```python
from build123d import *

# Parameters (mm, degrees)
BOSS_EXTRUDE1_DEPTH  = 19.05
BOSS_EXTRUDE2_DEPTH  = 6.35
M6_CLEARANCE_HOLE1_D = 6.4
FILLET1_R            = 1


with BuildPart() as part:
    # Sketch1 → Boss-Extrude1 (new body)
    with BuildSketch(Plane(origin=(0, 0, 0), x_dir=(1, 0, 0), z_dir=(0, 1, 0))):
        with BuildLine():
            Line((-7.566372975, 10.2), (7.566372975, 10.2))
            ThreePointArc((7.566372975, 10.2), (12.7, 0), (7.566372975, -10.2))
            Line((7.566372975, -10.2), (-7.566372975, -10.2))
            ThreePointArc((-7.566372975, -10.2), (-12.7, 0), (-7.566372975, 10.2))
        make_face()
    extrude(amount=BOSS_EXTRUDE1_DEPTH)

    # Sketch1<4> → Boss-Extrude2 (add)
    with BuildSketch(Plane(origin=(0, 0, 0), x_dir=(1, 0, 0), z_dir=(0, 1, 0))):
        with BuildLine():
            Line((13.919410907, 37.5), (-13.919410907, 37.5))
            ThreePointArc((-13.919410907, 37.5), (-28.284271247, 28.284271247), (-37.5, 13.919410907))
            Line((-37.5, 13.919410907), (-37.5, -13.919410907))
            ThreePointArc((-37.5, -13.919410907), (-28.284271247, -28.284271247), (-13.919410907, -37.5))
            Line((-13.919410907, -37.5), (13.919410907, -37.5))
            ThreePointArc((13.919410907, -37.5), (28.284271247, -28.284271247), (37.5, -13.919410907))
            Line((37.5, -13.919410907), (37.5, 13.919410907))
            ThreePointArc((37.5, 13.919410907), (28.284271247, 28.284271247), (13.919410907, 37.5))
        make_face()
    extrude(amount=-BOSS_EXTRUDE2_DEPTH)

    # M6 Clearance Hole1 (through all)
    with Locations(Plane(origin=(-30, 0, 0), x_dir=(0, 0, 1), z_dir=(0, 1, 0))):
        with Locations((0, 0), (-25.980762114, 15), (-25.980762114, 45), (0, 60), (25.980762114, 45), (25.980762114, 15)):
            Hole(M6_CLEARANCE_HOLE1_D / 2)

    # Fillet1
    fillet1_edges = [part.edges().sort_by_distance(p)[0] for p in [
        (-7.566372975, 9.525, 10.2),
        (-7.566372975, 9.525, -10.2),
        (7.566372975, 9.525, -10.2),
        (7.566372975, 9.525, 10.2),
    ]]
    fillet(fillet1_edges, radius=FILLET1_R)


solid = part.part
```
Model file for the job. Use its own axes, mm. A direction names the side the tool comes from. Coordinates: 2 decimals unless noted, no trailing zeros. Write each loop counter-clockwise with the first axis right and the second up, starting at its lowest first coordinate (ties: lowest second). Pieces come first, ordered by that corner, then holes. Notation, with made-up numbers: (37.5, 37.5) - (83.5, 37.5) arc R17 ccw to (83.5, 43.5) - close; hole circle Ø9 at (42.25, 16). An arc over 180 degrees is marked (long way). One line per item, written item: value. Start each with the question number.
1. Tool access for faces 4 (the cylindrical face through (12.7, 9.4, -0.2)), 5 (the cylindrical face through (-12.7, 9.4, 0.2)), 6 (the flat face through (0, 9, 10.2)), 7 (the flat face through (0, 9, -10.2)): list every direction of +Z, -Z, +X, -X, +Y, -Y with a clear straight run to the whole face (end or side of a thin tool).
2. Flat gauge pins, fed straight in: pin 1 (4.5 mm diameter, centred on x = 3, y = 12, fed in from -Z); pin 2 (8.5 mm diameter, centred on x = -15, z = -25.98, fed in from +Y); pin 3 (6 mm diameter, centred on y = 2.5, z = 27.5, fed in from +X). Where does each tip first touch, or does it go through?
3. Mould opens along X. For faces 1 (the cylindrical face through (28.454, -3.131, -28.113)), 2 (the flat face through (-37.5, -3, 0)), 3 (the cylindrical face through (-26.827, -3.219, 0.417)) say: released by +X, released by -X, zero draft, split by the parting line, or undercut.
4. Slice it at C-C (x = -15). Write the cut outline in (y, z), plus the area to 3 significant figures.
5. Probe line 1 (X direction, y = -3.75, z = 0); line 2 (Y direction, x = 25, z = 10); line 3 (Z direction, x = 7, y = 1). List the from-to ranges inside material, lowest first. Write a range as from..to.
6. Slice it at A-A (z = 0). Write the cut outline in (x, y), plus the area to 3 significant figures.
7. Slice it at D-D (y = 2.5). Write the cut outline in (x, z), plus the area to 3 significant figures.
8. Slice it at B-B (y = -3.5). Write the cut outline in (x, z), plus the area to 3 significant figures.
Answers below:
1. face 4: +X, +Y
1. face 5: -X, +Y
1. face 6: +Z, +X, -X, +Y
1. face 7: -Z, +X, -X, +Y
2. pin 1: stops at z = -10.2
2. pin 2: stops at y = 0
2. pin 3: stops at x = 30.53
3. face 1: released by +X
3. face 2: released by -X
3. face 3: undercut
4. outline: (-6.35, -37.08) - (0, -37.08) - (0, -29.18) - (-6.35, -29.18) - close; (-6.35, -22.78) - (0, -22.78) - (0, 22.78) - (-6.35, 22.78) - close; (-6.35, 29.18) - (0, 29.18) - (0, 37.08) - (-6.35, 37.08) - close
4. area: 390 mm^2
5. line 1: x = -37.5..-33.2, -26.8..26.8, 33.2..37.5
5. line 2: y = -6.35..0
5. line 3: z = -10.2..10.2
6. outline: (-37.5, -6.35) - (-33.2, -6.35) - (-33.2, 0) - (-37.5, 0) - close; (-26.8, -6.35) - (26.8, -6.35) - (26.8, 0) - (12.7, 0) - (12.7, 19.05) - (-12.7, 19.05) - (-12.7, 0) - (-26.8, 0) - close; (33.2, -6.35) - (37.5, -6.35) - (37.5, 0) - (33.2, 0) - close
6. area: 879 mm^2
7. outline: (-7.85, -9.99) arc R1 ccw to (-7.23, -10.2) - (7.23, -10.2) arc R1 ccw to (7.85, -9.99) arc R12.7 ccw to (7.85, 9.99) arc R1 ccw to (7.23, 10.2) - (-7.23, 10.2) arc R1 ccw to (-7.85, 9.99) arc R12.7 ccw to start
7. area: 455 mm^2
8. outline: (-37.5, -13.92) arc R40 ccw to (-13.92, -37.5) - (13.92, -37.5) arc R40 ccw to (37.5, -13.92) - (37.5, 13.92) arc R40 ccw to (13.92, 37.5) - (-13.92, 37.5) arc R40 ccw to (-37.5, 13.92) - close; hole circle Ø6.4 at (-30, 0); hole circle Ø6.4 at (-15, -25.98); hole circle Ø6.4 at (-15, 25.98); hole circle Ø6.4 at (15, -25.98); hole circle Ø6.4 at (15, 25.98); hole circle Ø6.4 at (30, 0)
8. area: 4,650 mm^2
